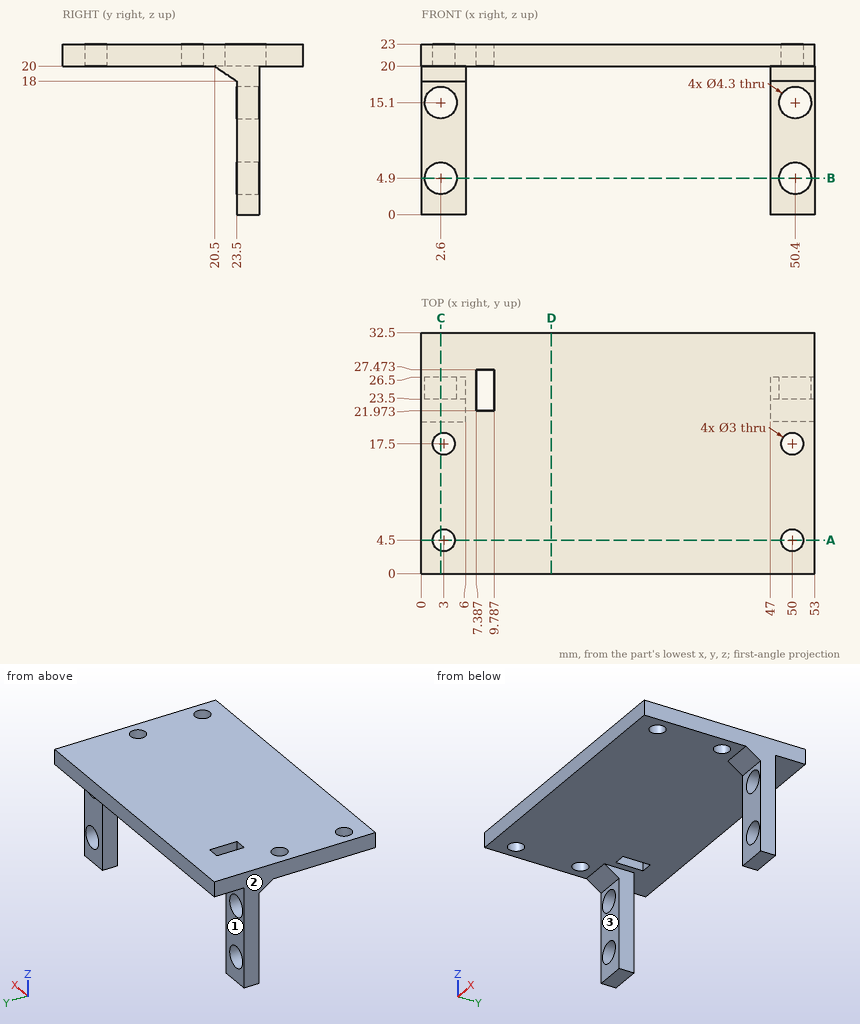
Verification items for this drawing (mm, ordinates from the low corner). A direction names the side the tool comes from. Give positions to 0.01 mm unless a question says otherwise; leave off trailing zeros. Loops run counter-clockwise (first coordinate to the right, second up) from the corner with the lowest first, then second, coordinate; pieces in that order, holes last. Notation, with made-up numbers: M 62.25,32 L 102.25,32 A23 ccw 102.25,70 Z; hole C 29,32.25 d4. An arc over 180 degrees is marked long. Answer as a JSON object with one key per item and string values. Group by question number.
Item 1: Sectioned sample at C-C on x = 2.6. Record the boundary of the cut face in (y, z), plus the area to 3 significant figures.
Item 2: Sectioned sample at B-B on z = 4.9. Record the boundary of the cut face in (x, y).
Item 3: Sectioned sample at D-D on x = 17.5. Record the boundary of the cut face in (y, z).
Item 4: Gauge pin test, flat ends, axial feed: pin 1 (5 mm diameter, centred on x = 2.5, z = 8.5, fed in from +Y); pin 2 (5 mm diameter, centred on x = 1.5, z = 13.5, fed in from -Y); pin 3 (1 mm diameter, centred on x = 26.5, y = 19, fed in from -Z); pin 4 (4 mm diameter, centred on x = 2.6, z = 15.1, fed in from +Y). Record the tip position at first contact, or that the pin passes through.
Item 5: Material ranges on L1, parallel to Y at x = 3, z = 20.85; L2, parallel to X at y = 25.5, z = 4.9; L3, parallel to Z at x = 50, y = 24, recorded low to high.
Item 6: Access from +Z, -Z, +X, -X, +Y, -Y to the whole of each face (thin tool, end or side, straight path). Record for the marked faces 1, 2 and 3.
Item 7: Sectioned sample at A-A on y = 4.5. Record the boundary of the cut face in (x, z), plus the area to 3 significant figures.
Findings below:
{
 "1": {"outline": "M 0,20 L 3.05,20 L 3.05,23 L 0,23 Z; M 5.95,20 L 16.05,20 L 16.05,23 L 5.95,23 Z; M 18.95,20 L 20.5,20 L 23.5,18 L 23.5,17.25 L 26.5,17.25 L 26.5,20 L 32.5,20 L 32.5,23 L 18.95,23 Z; M 23.5,0 L 26.5,0 L 26.5,2.75 L 23.5,2.75 Z; M 23.5,7.05 L 26.5,7.05 L 26.5,12.95 L 23.5,12.95 Z", "area": "117 mm2"},
 "2": {"outline": "M 0,23.5 L 0.45,23.5 L 0.45,26.5 L 0,26.5 Z; M 4.75,23.5 L 6,23.5 L 6,26.5 L 4.75,26.5 Z; M 47,23.5 L 48.25,23.5 L 48.25,26.5 L 47,26.5 Z; M 52.55,23.5 L 53,23.5 L 53,26.5 L 52.55,26.5 Z"},
 "3": {"outline": "M 0,20 L 32.5,20 L 32.5,23 L 0,23 Z"},
 "4": {"pin 1": "y = 26.5", "pin 2": "y = 23.5", "pin 3": "z = 20", "pin 4": "through"},
 "5": {"L1": "0 to 3, 6 to 16, 19 to 32.5", "L2": "0 to 0.45, 4.75 to 6, 47 to 48.25, 52.55 to 53", "L3": "0 to 2.79, 7.01 to 12.99, 17.21 to 23"},
 "6": {"face 1": "-Z, +X, -X, +Y", "face 2": "+Z, -Z, -X, +Y, -Y", "face 3": "-Z, +X, -X, -Y"},
 "7": {"outline": "M 0,20 L 1.5,20 L 1.5,23 L 0,23 Z; M 4.5,20 L 48.5,20 L 48.5,23 L 4.5,23 Z; M 51.5,20 L 53,20 L 53,23 L 51.5,23 Z", "area": "141 mm2"}
}
